Check sheet for the modelled part. Datum: model origin and axes. Units: mm. Face numbers are marked on the shaded views. A direction names the side the tool comes from. Give positions to 0.01 mm unless a question says otherwise; leave off trailing zeros. Loops run counter-clockwise (first coordinate to the right, second up) from the corner with the lowest first, then second, coordinate; pieces in that order, holes last. Notation, with made-up numbers: M 47,28.25 L 70,28.25 A21 ccw 70,67.25 Z; hole C 72.25,54.5 d8. An arc over 180 degrees is marked long. Put each result on its own line as item: value. Start each with the question number.
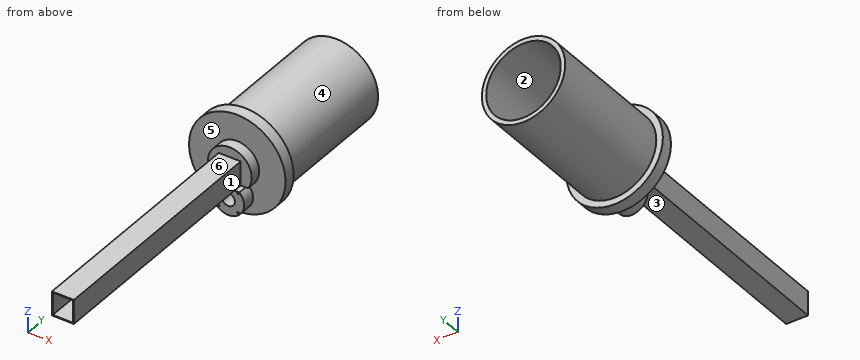
Autodesk Inventor part; units mm, degrees
ref_plane "YZ Plane" through (0, 0, 0) normal (1, 0, 0) x (0, 1, 0)
ref_plane "XZ Plane" through (0, 0, 0) normal (0, 1, 0) x (-1, 0, 0)
ref_plane "XY Plane" through (0, 0, 0) normal (0, 0, 1) x (1, 0, 0)
sketch "Sketch1" plane through (0, 0, 0) normal (0, 1, 0) x (-1, 0, 0)
  circle A0 centre (0, 0) radius 110
  circle A1 centre (0, 0) radius 95
  dimension "d0" = 220
  dimension "d1" = 190
extrude "Extrusion1" add sketch "Sketch1" along normal blind 330 contours A1
extrude "Extrusion2" add sketch "Sketch1" along normal blind 27
sketch "Sketch2" plane through (0, 330, 0) normal (0, 1, 0) x (1, 0, 0)
  circle A0 centre (0, 0) radius 85
  dimension "d6" = 170
extrude "Extrusion3" cut sketch "Sketch2" against normal blind 300
sketch "Sketch3" plane through (0, 0, 0) normal (0, -1, 0) x (1, 0, 0)
  arc A0 (-25.4, -40.4884) -> (25.4, -40.4884) centre (0, -66) ccw
  circle A1 centre (0, 0) radius 110
  line L0 (25.4, -40.4884) -> (-25.4, -40.4884)
  line L1 (25, -27.5) -> (-25, -27.5)
  line L2 (-25, -27.5) -> (-25, 27.5)
  line L3 (-25, 27.5) -> (25, 27.5)
  line L4 (25, 27.5) -> (25, -27.5)
  line L5 (25, -27.5) -> (-25, 27.5) construction
  line L6 (-25, -27.5) -> (25, 27.5) construction
  arc A2 (41.7582, -27.5) -> (-41.7582, -27.5) centre (0, 0) ccw
  line L7 (25, -27.5) -> (41.7582, -27.5)
  line L8 (-25, -27.5) -> (-41.7582, -27.5)
  dimension "d9" = 72
  dimension "d10" = 66
  dimension "d11" = 50
  dimension "d12" = 55
  dimension "d13" = 100
extrude "Extrusion4" add sketch "Sketch3" along normal blind 25 contours L1 L2 L3 L4 | L4 L3 L2 L8 A2 L7
extrude "Extrusion5" add sketch "Sketch3" along normal blind 580 contours L1 L2 L3 L4
extrude "Extrusion6" add sketch "Sketch3" along normal blind 30 contours L0 A0
sketch "Sketch4" plane through (0, -580, 0) normal (0, -1, 0) x (1, 0, 0)
  line L0 (-25, 27.5) -> (25, 27.5)
  line L1 (-25, -27.5) -> (25, -27.5)
  line L2 (25, -27.5) -> (25, 27.5)
  line L3 (25, 27.5) -> (-25, 27.5)
  line L4 (-25, 27.5) -> (-25, -27.5)
  line L5 (-25, -27.5) -> (25, 27.5) construction
  line L6 (25, -27.5) -> (-25, 27.5) construction
  line L7 (23, 25.5) -> (23, -25.5)
  line L8 (23, -25.5) -> (-23, -25.5)
  line L9 (-23, -25.5) -> (-23, 25.5)
  line L10 (-23, 25.5) -> (23, 25.5)
  point P0 (0, 0)
  dimension "d20" = 2
extrude "Extrusion7" cut sketch "Sketch4" against normal through all contours L7 L8 L9 L10
sketch "Sketch5" plane through (0, -30, 0) normal (0, -1, 0) x (1, 0, 0)
  arc A0 (-25.4, -40.4884) -> (25.4, -40.4884) centre (0, -66) ccw
  circle A1 centre (0, -66) radius 36
  line L0 (-25.4, -40.4884) -> (25.4, -40.4884)
  line L1 (25.4, -40.4884) -> (-25.4, -40.4884)
  circle A2 centre (0, -66) radius 32.5
  line L2 (22.225, -43.775) -> (-22.225, -43.775)
  line L3 (-22.225, -43.775) -> (-22.225, -88.225)
  line L4 (-22.225, -88.225) -> (22.225, -88.225)
  line L5 (22.225, -88.225) -> (22.225, -43.775)
  line L6 (22.225, -43.775) -> (-22.225, -88.225) construction
  line L7 (-22.225, -43.775) -> (22.225, -88.225) construction
  circle A3 centre (-22.225, -88.225) radius 2.25
  circle A4 centre (-22.225, -43.775) radius 2.25
  circle A5 centre (22.225, -88.225) radius 2.25
  circle A6 centre (22.225, -43.775) radius 2.25
  circle A7 centre (0, -66) radius 15
  point P0 (0, 0)
  dimension "d23" = 65
  dimension "d24" = 44.45
  dimension "d25" = 4.5
  dimension "d26" = 4.5
  dimension "d27" = 4.5
  dimension "d28" = 4.5
  dimension "d29" = 30
extrude "Extrusion8" cut sketch "Sketch5" against normal blind 10 contours A4 L2 L3 A2 | A2 A4 | A6 A2 | A2 A6 L5 L2 | A4 L3 L2 | L2 L5 A6 | A3 L3 L4 A2 | A2 A3 | A3 L4 L3 | A5 A2 | A2 A5 L4 L5 | L5 L4 A5
extrude "Extrusion9" cut sketch "Sketch5" against normal through all contours A7
properties part number "Plunger"
Q1. Section check D-D, the plane z = -66. Record the cut outline in (x, y), then the cut area to 3 significant figures.
Q2. Section check C-C, the plane y = -49. Record the cut outline in (x, z).
Q3. Section check A-A, the plane z = 0. Record the cut outline in (x, y), then the cut area to 3 significant figures.
Q4. Section check B-B, the plane x = 0. Give the number of separate pieces and of enclosed holes in the cut face, then the cut area to 3 significant figures.
Q5. Thickness scan on line 1 along Z through (x, y) = (0, 9); line 2 along Z through (x, y) = (-1, 286.5); line 3 along Y through (x, z) = (50, 54). Record the ranges inside material, lowest first. Write a range as [from, to].
Q6. Depth check by flat-ended pin: P1, Ø4, axis at y = -387.5, z = 11.5, coming from the +X side; P2, Ø3.5, axis at x = -22.225, z = -43.775, coming from the -Y side; P3, Ø15, axis at x = -9.5, y = -12, coming from the +Z side. Enter the tip coordinate at first touch or a pass-through.
Q7. Mould release check, pull along X, two halves, no side actions. Record for the marked faces 1, 2, 3 and 4: pulls with the +X half, pulls with the -X half, needs draft (parallel to the pull), parting line crosses it, or undercut.
Q8. Access from +Z, -Z, +X, -X, +Y, -Y to the whole of each face (thin tool, end or side, straight path). Record for the marked faces 5 and 6.
Found:
1. outline: M -88,0 L -36,0 L -36,-30 L -15,-30 L -15,30 L -53.56,30 L -53.56,330 L -68.33,330 L -68.33,27 L -88,27 Z; M 15,-30 L 36,-30 L 36,0 L 88,0 L 88,27 L 68.33,27 L 68.33,330 L 53.56,330 L 53.56,30 L 15,30 Z
1. area: 14,400 mm^2
2. outline: M -25,-27.5 L 25,-27.5 L 25,27.5 L -25,27.5 Z; hole M -23,-25.5 L 23,-25.5 L 23,25.5 L -23,25.5 Z
3. outline: M -110,0 L -50,0 L -50,-25 L -25,-25 L -25,-580 L -23,-580 L -23,30 L -85,30 L -85,330 L -95,330 L -95,27 L -110,27 Z; M 23,-580 L 25,-580 L 25,-25 L 50,-25 L 50,0 L 110,0 L 110,27 L 95,27 L 95,330 L 85,330 L 85,30 L 23,30 Z
3. area: 14,700 mm^2
4. separate pieces: 3
4. enclosed holes: 0
4. area: 13,900 mm^2
5. line 1: z = [-110, -81], [-51, -25.5], [25.5, 110]
5. line 2: z = [-94.99, -84.99], [84.99, 94.99]
5. line 3: y = [0, 30]
6. P1: stops at x = 25
6. P2: stops at y = -20
6. P3: stops at z = 49.96
7. face 1: pulls with the +X half
7. face 2: undercut
7. face 3: needs draft
7. face 4: parting line crosses it
8. face 5: -Y
8. face 6: +Z, +X, -X, -Y
